Verification items for this drawing (mm, ordinates from the low corner). A direction names the side the tool comes from. Coordinates: 2 decimals unless noted, no trailing zeros. Order: outer loops, then holes, each group sorted by start corner. A loop starts at its lowest first (then second) coordinate and runs counter-clockwise, first axis right, second up. Notation, with made-up numbers: M 37,-21.5 L 62,-21.5 A20 cw 62,-17.5 Z; hole C 86.5,-29.5 d3. An arc over 180 degrees is marked long. Write item = value, one per line.
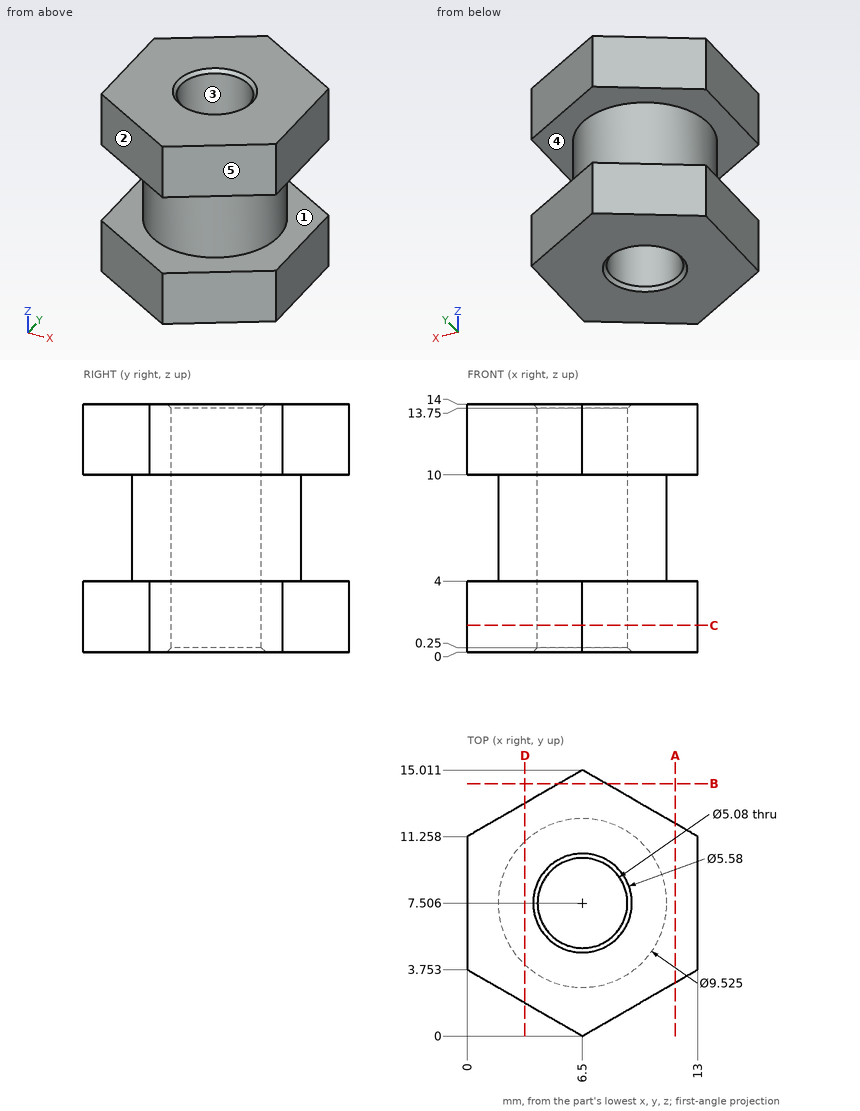
Item 1: Tool access check on the marked faces 4 and 5. Record the directions out of +Z, -Z, +X, -X, +Y, -Y that give a thin tool (end or side, any length) a straight path to the whole face; none if there is none.
Report:
face_4 = none
face_5 = +Z, -Z, +X, -Y
Item 2: Sectioned sample at D-D, the plane x = 3.25. Enter the section's corners in (y, z) (1 decimal), then the cut area to 3 significant figures.
Report:
outline = M 1.9,0 L 13.1,0 L 13.1,4 L 11,4 L 11,10 L 13.1,10 L 13.1,14 L 1.9,14 L 1.9,10 L 4,10 L 4,4 L 1.9,4 Z
area = 132 mm^2
Item 3: Sectioned sample at B-B, the plane y = 14.25. Enter the section's corners in (x, z).
Report:
outline = M 5.18,0 L 7.82,0 L 7.82,4 L 5.18,4 Z; M 5.18,10 L 7.82,10 L 7.82,14 L 5.18,14 Z
Item 4: Scan lines: L1, parallel to Y at x = 6.5, z = 8.75 (1 decimal); L2, parallel to Z at x = 6, y = 13.25; L3, parallel to X at y = 7.5, z = 12.5. Record each from-to range of solid material in increasing order. Write a range as from..to.
Report:
L1 = 2.7..5, 10..12.3
L2 = 0..4, 10..14
L3 = 0..3.96, 9.04..13
Item 5: Release check for a two-part mould opening along Y. For the marked faces 1, 2 and 3 record: pulls with the +Y half, pulls with the -Y half, needs draft (parallel to the pull), parting line crosses it, or undercut.
Report:
face_1 = needs draft
face_2 = pulls with the -Y half
face_3 = undercut
Item 6: Sectioned sample at C-C, the plane z = 1.5. Enter the section's corners in (x, y) (1 decimal), then the cut area to 3 significant figures.
Report:
outline = M 0,3.8 L 6.5,0 L 13,3.8 L 13,11.3 L 6.5,15 L 0,11.3 Z; hole C 6.5,7.5 d5.1
area = 126 mm^2
Item 7: Gauge pin test, flat ends, axial feed: pin 1 (6.5 mm diameter, centred on x = 6.5, y = 7.51, fed in from -Z); pin 2 (2 mm diameter, centred on x = 5, z = 2, fed in from +Y); pin 3 (3 mm diameter, centred on y = 2, z = 7.5, fed in from -X) (1 decimal); pin 4 (1 mm diameter, centred on y = 10.5, z = 8.5, fed in from -X). Record the tip position at first contact, or that the pin passes through.
Report:
pin_1 = 0
pin_2 = 14.72
pin_3 = 3.9
pin_4 = 2.44
Item 8: Sectioned sample at A-A, the plane x = 11.75. Enter the section's corners in (y, z).
Report:
outline = M 3.03,0 L 11.98,0 L 11.98,4 L 3.03,4 Z; M 3.03,10 L 11.98,10 L 11.98,14 L 3.03,14 Z
